The model under review builds one solid part; all positions refer to its coordinate system, in mm. A direction names the side the tool comes from. Coordinates: 2 decimals unless noted, no trailing zeros. Loops run counter-clockwise (first coordinate to the right, second up) from the corner with the lowest first, then second, coordinate; pieces in that order, holes last. Notation, with made-up numbers: (69, -2.75) - (104, -2.75) arc R28 cw to (104, 27.25) - close; hole circle Ø5 at (20, 69). An arc over 180 degrees is marked (long way). One line per item, written item: value. Start each with the question number.
1. To check wall thickness, follow line 1 (Z direction, x = -8, y = 3.6); line 2 (X direction, y = 4.5, z = 27); line 3 (Z direction, x = -10, y = 4.7). State the ranges of each line that lie inside material, in increasing order.
2. For faces 4 (the face through (-8, 3, 34)), 5 (the face through (-16, 2, 30)), list the 3-axis set-ups (+Z, -Z, +X, -X, +Y, -Y) from which the entire face can be reached by the end or side of a thin tool; tool diameter is ignored.
3. We need section B-B, the plane x = -8. Give the boundary of the cut face in (y, z), then the cut area to 3 significant figures.
4. Insertion check: P1, Ø8, axis at x = -8, z = 51, coming from the -Y side. The pin has a flat end and moves straight along its axis. Give the tip position at first contact, or say it passes through.
5. Mouldability with a two-part tool opening along X and no side actions: class faces 1 (the face through (-10.5, 3, 30)), 2 (the face through (0, 2, 30)), 3 (the face through (-11, 0, 30)) as +X half, -X half, draft (parallel to the pull), parting line (faces both ways), or undercut.
6. We need section C-C, the plane y = 3.55. Give the boundary of the cut face in (x, z), then the cut area to 3 significant figures.
7. We need section A-A, the plane z = 51. Give the boundary of the cut face in (x, y).
Autodesk Inventor part; units mm, degrees
ref_plane "YZ Plane" through (0, 0, 0) normal (1, 0, 0) x (0, 1, 0)
ref_plane "XZ Plane" through (0, 0, 0) normal (0, 1, 0) x (-1, 0, 0)
ref_plane "XY Plane" through (0, 0, 0) normal (0, 0, 1) x (1, 0, 0)
sketch "Sketch1" plane through (0, 0, 0) normal (0, 1, 0) x (-1, 0, 0)
  line L0 (0, 0) -> (16, 0)
  line L1 (16, 0) -> (16, 60)
  line L2 (16, 60) -> (0, 60)
  line L3 (0, 60) -> (0, 0)
  circle A0 centre (8, 51) radius 2.5
  circle A1 centre (8, 9) radius 2.5
  dimension "d2" = 60
  dimension "d3" = 16
  dimension "d4" = 8
  dimension "d5" = 5
  dimension "d6" = 9
  dimension "d7" = 8
  dimension "d8" = 9
  dimension "d9" = 5
extrude "Extrusion1" add sketch "Sketch1" along normal blind 5
sketch "Sketch2" plane through (0, 5, 0) normal (0, 1, 0) x (1, 0, 0)
  line L0 (-10.5, -26) -> (-5.5, -26)
  line L1 (-5.5, -26) -> (-5.5, -34)
  line L2 (-5.5, -34) -> (-10.5, -34)
  line L3 (-10.5, -34) -> (-10.5, -26)
  line L4 (-16, 0) -> (-16, -60)
  line L5 (-16, -60) -> (0, -60)
  line L6 (0, -60) -> (0, 0)
  dimension "d10" = 8
  dimension "d11" = 5
  dimension "d13" = 26
  dimension "d16" = 5.5
extrude "Extrusion2" cut sketch "Sketch2" against normal through all
properties part number "holder_sideblock"
Findings below:
1. line 1: 0 to 6.5, 11.5 to 26, 34 to 48.5, 53.5 to 60
1. line 2: -16 to -10.5, -5.5 to 0
1. line 3: 0 to 7.5, 10.5 to 26, 34 to 49.5, 52.5 to 60
2. face 4: +Y, -Y
2. face 5: +Z, -Z, -X, +Y, -Y
3. outline: (0, 0) - (5, 0) - (5, 6.5) - (0, 6.5) - close; (0, 11.5) - (5, 11.5) - (5, 26) - (0, 26) - close; (0, 34) - (5, 34) - (5, 48.5) - (0, 48.5) - close; (0, 53.5) - (5, 53.5) - (5, 60) - (0, 60) - close
3. area: 210 mm2
4. P1: y = 0
5. face 1: undercut
5. face 2: +X half
5. face 3: draft
6. outline: (-16, 0) - (0, 0) - (0, 60) - (-16, 60) - close; hole circle Ø5 at (-8, 9); hole (-10.5, 26) - (-5.5, 26) - (-5.5, 34) - (-10.5, 34) - close; hole circle Ø5 at (-8, 51)
6. area: 881 mm2
7. outline: (-16, 0) - (-10.5, 0) - (-10.5, 5) - (-16, 5) - close; (-5.5, 0) - (0, 0) - (0, 5) - (-5.5, 5) - close
